Can you work these out from the model? Positions are in its coordinate system, mm. Face numbers are marked on the shaded views. A direction names the side the tool comes from. Round coordinates to 2 decimals unless told otherwise and drop trailing zeros. Order: outer loops, then holes, each group sorted by start corner. A loop starts at its lowest first (then second) coordinate and runs counter-clockwise, first axis right, second up.
Q1. If I drill on line 1 (Y direction, x = 48, z = 10); line 2 (Z direction, x = 5, y = 3.3); line 3 (X direction, y = 3, z = 90), over which ranges is the centre line in solid material (lowest first)?
Q2. If we section it at A-A (x = 12): Please give me the cut outline in (y, z).
Q3. If we section it at C-C (z = 73): Please give me the cut outline in (x, y), plus the area to 3 significant figures.
Q4. If we section it at D-D (y = -13.25): Count the separate pieces of the cut face and the enclosed holes in it, plus the area to 3 significant figures.
Q5. For the marked faces 1, 2 and 3, which set-ups out of +Z, -Z, +X, -X, +Y, -Y let a thin tool reach every point of the face, with its end or its side?
Q6. If we section it at B-B (y = -8.75): Please give me the cut outline in (x, z).
Q7. Will these pins go through, and if not, where does the flat tip stop? P1, Ø4.5, axis at y = -14, z = 90.5, coming from the -X side; P2, Ø12, axis at x = 15.5, y = -15.5, coming from the +Z side; P3, Ø2.5, axis at y = -8, z = 39.5, coming from the -X side.
from build123d import *

# Parameters (mm, degrees)
CROQUIS1_W              = 50
CROQUIS1_H              = 100
CROQUIS1_R              = 1.6
SALIENTE_EXTRUIR1_DEPTH = 5
CROQUIS2_W              = 10
CROQUIS2_H              = 100
SALIENTE_EXTRUIR2_DEPTH = 25
CROQUIS3_R              = 1.6
CORTAR_EXTRUIR1_DEPTH   = 10
CORTAR_EXTRUIR2_DEPTH   = 1
REDONDEO1_R             = 8
CROQUIS5_W              = 60
CROQUIS5_H              = 15
SALIENTE_EXTRUIR3_DEPTH = 30
REDONDEO2_R             = 5
CROQUIS6_R              = 2.8
CORTAR_EXTRUIR3_DEPTH   = 1.5


with BuildPart() as part:
    # Croquis1 → Saliente-Extruir1 (new body)
    with BuildSketch(Plane(origin=(0, 0, 0), x_dir=(1, 0, 0), z_dir=(0, 1, 0))):
        with Locations((25, -50)):
            Rectangle(CROQUIS1_W, CROQUIS1_H)
        with Locations(Location((5, -10, 0), (0, 0, 270))):
            Circle(CROQUIS1_R, mode=Mode.SUBTRACT)
        with Locations(Location((5, -90, 0), (0, 0, 270))):
            Circle(CROQUIS1_R, mode=Mode.SUBTRACT)
    extrude(amount=SALIENTE_EXTRUIR1_DEPTH)

    # Croquis2 → Saliente-Extruir2 (add)
    with BuildSketch(Plane.XZ):
        with Locations((45, 50)):
            Rectangle(CROQUIS2_W, CROQUIS2_H)
    extrude(amount=SALIENTE_EXTRUIR2_DEPTH)

    # Croquis3 → Cortar-Extruir1 (cut)
    with BuildSketch(Plane.ZY.offset(-40)):
        with Locations((10, -13.25)):
            Circle(CROQUIS3_R)
        with Locations((90, -13.25)):
            Circle(CROQUIS3_R)
    extrude(amount=-CORTAR_EXTRUIR1_DEPTH, mode=Mode.SUBTRACT)

    # Croquis4 → Cortar-Extruir2 (cut)
    with BuildSketch(Plane.XZ):
        Polygon((3.325684219, 7.1), (6.674315781, 7.1), (8.348631561, 10), (6.674315781, 12.9), (3.325684219, 12.9), (1.651368439, 10), align=None)
        Polygon((3.325684219, 87.1), (6.674315781, 87.1), (8.348631561, 90), (6.674315781, 92.9), (3.325684219, 92.9), (1.651368439, 90), align=None)
    extrude(amount=-CORTAR_EXTRUIR2_DEPTH, mode=Mode.SUBTRACT)

    # Redondeo1
    redondeo1_edges = [part.edges().sort_by_distance(p)[0] for p in [
        (45, -25, 100),
        (45, -25, 0),
        (0, 2.5, 0),
        (0, 2.5, 100),
    ]]
    fillet(redondeo1_edges, radius=REDONDEO1_R)

    # Croquis5 → Saliente-Extruir3 (add)
    with BuildSketch(Plane.ZY.offset(-40)):
        with Locations((50, -7.5)):
            Rectangle(CROQUIS5_W, CROQUIS5_H)
    extrude(amount=SALIENTE_EXTRUIR3_DEPTH)

    # Redondeo2
    redondeo2_edges = [part.edges().sort_by_distance(p)[0] for p in [
        (40, 0, 10),
        (40, -7.5, 20),
        (25, 0, 20),
        (40, -15, 50),
        (40, -7.5, 80),
        (25, -15, 80),
        (25, 0, 80),
        (10, -15, 50),
        (10, 0, 50),
        (40, 0, 90),
    ]]
    fillet(redondeo2_edges, radius=REDONDEO2_R)

    # Croquis6 → Cortar-Extruir3 (cut)
    with BuildSketch(Plane.ZY.offset(-40)):
        with Locations((10, -13.25)):
            Circle(CROQUIS6_R)
        with Locations((90, -13.25)):
            Circle(CROQUIS6_R)
    extrude(amount=-CORTAR_EXTRUIR3_DEPTH, mode=Mode.SUBTRACT)


solid = part.part
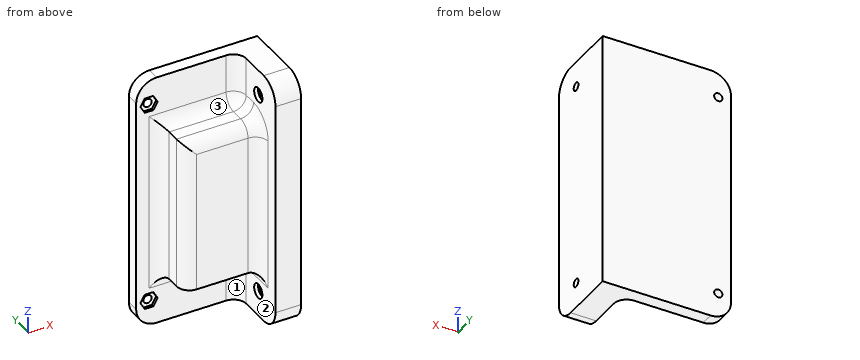
Solution:
1. line 1: y = -25 to -14.85, -11.65 to 5
1. line 2: z = 0.58 to 8.4, 11.6 to 88.4, 91.6 to 99.42
1. line 3: x = 0 to 3.4, 6.6 to 50
2. outline: (-14, 20) - (-5, 20) arc R5 cw to (0, 15) - (0, 0) - (5, 0) - (5, 100) - (0, 100) - (0, 85) arc R5 cw to (-5, 80) - (-10, 80) arc R5 ccw to (-14, 78) - close
3. outline: (0, 0) - (5, 0) arc R5 cw to (10, -5) - (10, -10) arc R5 ccw to (15, -15) - (35, -15) arc R5 cw to (40, -20) - (40, -25) - (50, -25) - (50, 5) - (0, 5) - close
3. area: 955 mm2
4. separate pieces: 3
4. enclosed holes: 0
4. area: 2,630 mm2
5. face 1: -Z, -X, -Y
5. face 2: -X, -Y
5. face 3: +Z, -X, -Y
6. outline: (10, 20) - (35, 20) arc R5 cw to (40, 15) - (40, 0) - (50, 0) - (50, 100) - (40, 100) - (40, 85) arc R5 cw to (35, 80) - (10, 80) - close
7. P1: stops at x = 40
7. P2: stops at z = 80
7. P3: stops at x = 10
